Part model, mm, in its own coordinate system. Round coordinates to 2 decimals unless told otherwise and drop trailing zeros. Write each loop counter-clockwise with the first axis right and the second up, starting at its lowest first coordinate (ties: lowest second). Pieces come first, ordered by that corner, then holes. Notation, with made-up numbers: M -16.5,7 L 8.5,7 A25 ccw 8.5,35 Z; hole C -37,38 d11. An arc over 180 degrees is marked long. Use a Markdown table: item, result. Add a question column.
1) Slice it at D-D on z = 1.45. Give the number of separate pieces and of enclosed holes in the cut face, plus the area to 3 significant figures.
2) Drop flat-ended pins along their axis: P1, Ø1, axis at y = 24.5, z = 1.5, coming from the +X side; P2, Ø0.6, axis at y = 26.5, z = 0.5, coming from the -X side. Give the stop position or say it passes through.
3) Slice it at C-C on x = 41. Write the cut outline in (y, z), plus the area to 3 significant figures.
4) Wall check: probe 1 along Y at (x, z) = (0, 0.6); probe 2 along X at (y, z) = (24, 1.75); probe 3 along Y at (x, z) = (2, 1.55). Give the ranges that are in metal, low to high.
5) Slice it at B-B on y = 0. Write the cut outline in (x, z), plus the area to 3 significant figures.
6) Slice it at A-A on x = 0. Write the cut outline in (y, z), plus the area to 3 significant figures.
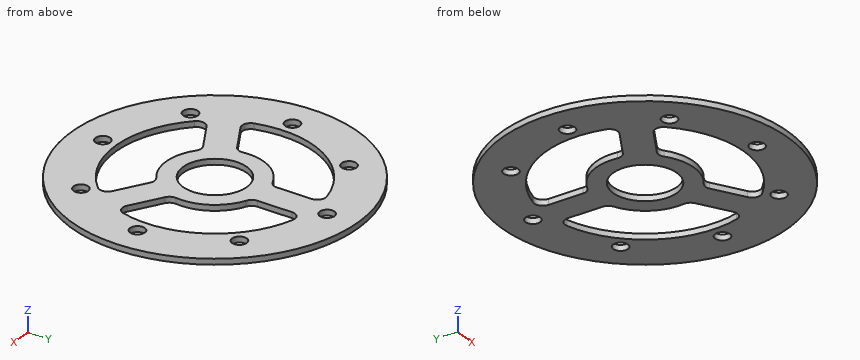
```python
from build123d import *

# Parameters (mm, degrees)
SKETCH_1_R      = 50.5
SKETCH_1_R_2    = 2.6
SKETCH_1_R_3    = 35
EXTRUDE_1_DEPTH = 2
EXTRUDE_START   = -2
SKETCH_2_R      = 11.25
EXTRUDE_3_DEPTH = 2
FILLET_1_R      = 3


with BuildPart() as part:
    # 草图1 → 凸台-拉伸1 (new body)
    with BuildSketch(Plane.XY):
        Circle(SKETCH_1_R)
        with Locations((0, 40)):
            Circle(SKETCH_1_R_2, mode=Mode.SUBTRACT)
        Circle(SKETCH_1_R_3, mode=Mode.SUBTRACT)
        with Locations((28.284271247, 28.284271247)):
            Circle(SKETCH_1_R_2, mode=Mode.SUBTRACT)
        with Locations((40, 0)):
            Circle(SKETCH_1_R_2, mode=Mode.SUBTRACT)
        with Locations((28.284271247, -28.284271247)):
            Circle(SKETCH_1_R_2, mode=Mode.SUBTRACT)
        with Locations((0, -40)):
            Circle(SKETCH_1_R_2, mode=Mode.SUBTRACT)
        with Locations((-28.284271247, -28.284271247)):
            Circle(SKETCH_1_R_2, mode=Mode.SUBTRACT)
        with Locations((-40, 0)):
            Circle(SKETCH_1_R_2, mode=Mode.SUBTRACT)
        with Locations((-28.284271247, 28.284271247)):
            Circle(SKETCH_1_R_2, mode=Mode.SUBTRACT)
    extrude(amount=EXTRUDE_1_DEPTH)

    # 草图2 → 凸台-拉伸3 (add)
    with BuildSketch(Plane.XY.offset(2).offset(EXTRUDE_START)):
        with BuildLine():
            ThreePointArc((5, 34.641016151), (0, 35), (-5, 34.641016151))
            Line((-5, 34.641016151), (-5, 16.509466981))
            ThreePointArc((-5, 16.509466981), (-14.938938215, 8.625), (-16.797617809, -3.924606472))
            Line((-16.797617809, -3.924606472), (-32.5, -12.990381057))
            ThreePointArc((-32.5, -12.990381057), (-30.310889132, -17.5), (-27.5, -21.650635095))
            Line((-27.5, -21.650635095), (-11.797617809, -12.584860509))
            ThreePointArc((-11.797617809, -12.584860509), (0, -17.25), (11.797617809, -12.584860509))
            Line((11.797617809, -12.584860509), (27.5, -21.650635095))
            ThreePointArc((27.5, -21.650635095), (30.310889132, -17.5), (32.5, -12.990381057))
            Line((32.5, -12.990381057), (16.797617809, -3.924606472))
            ThreePointArc((16.797617809, -3.924606472), (14.938938215, 8.625), (5, 16.509466981))
            Line((5, 16.509466981), (5, 34.641016151))
        make_face()
        Circle(SKETCH_2_R, mode=Mode.SUBTRACT)
    extrude(amount=EXTRUDE_3_DEPTH)

    # 圆角1
    fillet_1_edges = [part.edges().sort_by_distance(p)[0] for p in [
        (-16.797617809, -3.924606472, 1),
        (-32.5, -12.990381057, 1),
        (-27.5, -21.650635095, 1),
        (-11.797617809, -12.584860509, 1),
        (11.797617809, -12.584860509, 1),
        (27.5, -21.650635095, 1),
        (32.5, -12.990381057, 1),
        (16.797617809, -3.924606472, 1),
        (5, 16.509466981, 1),
        (5, 34.641016151, 1),
        (-5, 34.641016151, 1),
        (-5, 16.509466981, 1),
    ]]
    fillet(fillet_1_edges, radius=FILLET_1_R)


solid = part.part
```
Entries:
| question | item | result |
|---|---|---|
| 1 | separate pieces | 1 |
| 1 | enclosed holes | 12 |
| 1 | area | 5,090 mm^2 |
| 2 | P1 | stops at x = 44.43 |
| 2 | P2 | stops at x = -43.17 |
| 3 | outline | M -29.48,0 L -2.4,0 L -2.4,2 L -29.48,2 Z; M 2.4,0 L 29.48,0 L 29.48,2 L 2.4,2 Z |
| 3 | area | 108 mm^2 |
| 4 | probe 1 | y = -50.5 to -42.6, -37.4 to -35, -17.25 to -11.25, 11.25 to 37.4, 42.6 to 50.5 |
| 4 | probe 2 | x = -44.43 to -25.48, -5 to 5, 25.48 to 44.43 |
| 4 | probe 3 | y = -50.46 to -41.66, -38.34 to -34.94, -17.13 to -11.07, 11.07 to 38.34, 41.66 to 50.46 |
| 5 | outline | M -50.5,0 L -42.6,0 L -42.6,2 L -50.5,2 Z; M -37.4,0 L -35,0 L -35,2 L -37.4,2 Z; M -17.25,0 L -11.25,0 L -11.25,2 L -17.25,2 Z; M 11.25,0 L 17.25,0 L 17.25,2 L 11.25,2 Z; M 35,0 L 37.4,0 L 37.4,2 L 35,2 Z; M 42.6,0 L 50.5,0 L 50.5,2 L 42.6,2 Z |
| 5 | area | 65.2 mm^2 |
| 6 | outline | M -50.5,0 L -42.6,0 L -42.6,2 L -50.5,2 Z; M -37.4,0 L -35,0 L -35,2 L -37.4,2 Z; M -17.25,0 L -11.25,0 L -11.25,2 L -17.25,2 Z; M 11.25,0 L 37.4,0 L 37.4,2 L 11.25,2 Z; M 42.6,0 L 50.5,0 L 50.5,2 L 42.6,2 Z |
| 6 | area | 101 mm^2 |
